from build123d import *

# Parameters (mm, degrees)
ESQUISSE1_R      = 15
ESQUISSE1_R_2    = 3.5
ESQUISSE1_R_3    = 2
ESQUISSE1_R_4    = 1.5
EXTRUSION1_DEPTH = 7
ESQUISSE2_R      = 4.5
ESQUISSE2_R_2    = 3.5
EXTRUSION2_DEPTH = 3
ESQUISSE3_R      = 6
EXTRUSION3_DEPTH = 4
ESQUISSE4_R      = 5
ESQUISSE4_R_2    = 3.5
EXTRUSION4_DEPTH = 0.5


with BuildPart() as part:
    # Esquisse1 → Extrusion1 (new body)
    with BuildSketch(Plane.XY):
        Circle(ESQUISSE1_R)
        Circle(ESQUISSE1_R_2, mode=Mode.SUBTRACT)
        with Locations((10.608811196, -6.125)):
            Circle(ESQUISSE1_R_3, mode=Mode.SUBTRACT)
        with Locations((0, 12.25)):
            Circle(ESQUISSE1_R_3, mode=Mode.SUBTRACT)
        with Locations((-10.608811196, -6.125)):
            Circle(ESQUISSE1_R_3, mode=Mode.SUBTRACT)
        with Locations((-6.92820323, 4)):
            Circle(ESQUISSE1_R_4, mode=Mode.SUBTRACT)
        with Locations((6.92820323, 4)):
            Circle(ESQUISSE1_R_4, mode=Mode.SUBTRACT)
        with Locations((0, -8)):
            Circle(ESQUISSE1_R_4, mode=Mode.SUBTRACT)
    extrude(amount=EXTRUSION1_DEPTH)

    # Esquisse2 → Extrusion2 (add)
    with BuildSketch(Plane.XY.offset(7)):
        Circle(ESQUISSE2_R)
        Circle(ESQUISSE2_R_2, mode=Mode.SUBTRACT)
    extrude(amount=EXTRUSION2_DEPTH)

    # Esquisse3 → Extrusion3 (cut)
    with BuildSketch(Plane(origin=(0, 0, 0), x_dir=(-1, 0, 0), z_dir=(0, 0, -1))):
        Circle(ESQUISSE3_R)
    extrude(amount=-EXTRUSION3_DEPTH, mode=Mode.SUBTRACT)

    # Esquisse4 → Extrusion4 (cut)
    with BuildSketch(Plane(origin=(0, 0, 4), x_dir=(-1, 0, 0), z_dir=(0, 0, -1))):
        Circle(ESQUISSE4_R)
        Circle(ESQUISSE4_R_2, mode=Mode.SUBTRACT)
    extrude(amount=-EXTRUSION4_DEPTH, mode=Mode.SUBTRACT)


solid = part.part
Geometry: final body of the model. Coordinates: model frame, mm. A direction names the side the tool comes from. Give positions to 0.01 mm unless a question says otherwise; leave off trailing zeros. Write each loop counter-clockwise with the first axis right and the second up, starting at its lowest first coordinate (ties: lowest second). Pieces come first, ordered by that corner, then holes.
(1) Access query for faces 1 (the flat face through (0, -4, 10)), 2 (the cylindrical face through (1.08, -4.88, 4.25)), 3 (the flat face through (-4, -3, 7)). Directions: +Z, -Z, +X, -X, +Y, -Y. A direction counts if a zero-diameter tool reaches every point of the face in a straight line with its end or side. Return the directions, or none.
(2) Ray query, line 1 (Y direction, x = 0, z = 2.55); line 2 (Y direction, x = 0.5, z = 5.25); line 3 (Z direction, x = 3.25, y = 11.75). Return the intervals inside material, ascending.
(3) Cut plane D-D, the plane y = 4. Return loops of the section in (x, z), then the cut area to 3 significant figures.
(4) Cut plane B-B, the plane x = 0. Return loops of the section in (y, z).
(5) First-contact query: P1, Ø3.5, axis at x = 1.5, y = -2, coming from the -Z side; P2, Ø5, axis at x = -10.61, y = -6.12, coming from the +Z side; P3, Ø5, axis at x = 0, y = -0.5, coming from the -Z side; P4, Ø1.5, axis at y = 4, z = 1, coming from the +X side. Flat tips, straight axial feed; report the tip coordinate or a pass-through.
(6) Cut plane A-A, the plane y = 0. Return loops of the section in (x, z).
(7) Mould query, pull axis Y, two halves, no side actions, for faces 4 (the flat face through (6.5, 0.2, 0)), 5 (the cylindrical face through (-14.985, 0.66, 3.451)), 6 (the cylindrical face through (3.233, -1.341, 7.212)). Classes: released by +Y, released by -Y, zero draft, split by the parting line, or undercut.
(8) Cut plane C-C, the plane x = 11.75. Return loops of the section in (y, z).
Values follow:
1. face 1: +Z, +X, -X, +Y, -Y
1. face 2: -Z
1. face 3: +Z
2. line 1: y = -15 to -9.5, -6.5 to -6, 6 to 10.25, 14.25 to 15
2. line 2: y = -14.99 to -9.41, -6.59 to -3.46, 3.46 to 10.31, 14.19 to 14.99
2. line 3: z = 0 to 7
3. outline: (-14.46, 0) - (-8.43, 0) - (-8.43, 7) - (-14.46, 7) - close; (-5.43, 0) - (-4.47, 0) - (-4.47, 4) - (-3, 4) - (-3, 4.5) - (3, 4.5) - (3, 4) - (4.47, 4) - (4.47, 0) - (5.43, 0) - (5.43, 7) - (2.06, 7) - (2.06, 10) - (-2.06, 10) - (-2.06, 7) - (-5.43, 7) - close; (8.43, 0) - (14.46, 0) - (14.46, 7) - (8.43, 7) - close
3. area: 134 mm2
4. outline: (-15, 0) - (-9.5, 0) - (-9.5, 7) - (-15, 7) - close; (-6.5, 0) - (-6, 0) - (-6, 4) - (-5, 4) - (-5, 4.5) - (-3.5, 4.5) - (-3.5, 10) - (-4.5, 10) - (-4.5, 7) - (-6.5, 7) - close; (3.5, 4.5) - (5, 4.5) - (5, 4) - (6, 4) - (6, 0) - (10.25, 0) - (10.25, 7) - (4.5, 7) - (4.5, 10) - (3.5, 10) - close; (14.25, 0) - (15, 0) - (15, 7) - (14.25, 7) - close
5. P1: stops at z = 4.5
5. P2: stops at z = 7
5. P3: passes through
5. P4: stops at x = 14.64
6. outline: (-15, 0) - (-6, 0) - (-6, 4) - (-5, 4) - (-5, 4.5) - (-3.5, 4.5) - (-3.5, 10) - (-4.5, 10) - (-4.5, 7) - (-15, 7) - close; (3.5, 4.5) - (5, 4.5) - (5, 4) - (6, 4) - (6, 0) - (15, 0) - (15, 7) - (4.5, 7) - (4.5, 10) - (3.5, 10) - close
7. face 4: zero draft
7. face 5: split by the parting line
7. face 6: undercut
8. outline: (-9.32, 0) - (-7.77, 0) - (-7.77, 7) - (-9.32, 7) - close; (-4.48, 0) - (9.32, 0) - (9.32, 7) - (-4.48, 7) - close
